```python
from build123d import *

# Parameters (mm, degrees)
SKETCH1_W           = 40
SKETCH1_H           = 60
BOSS_EXTRUDE1_DEPTH = 20
SKETCH2_R           = 15
CUT_EXTRUDE1_DEPTH  = 9
SKETCH3_R           = 2
CUT_EXTRUDE2_DEPTH  = 32
SKETCH4_W           = 15
SKETCH4_H           = 15
CUT_EXTRUDE3_DEPTH  = 9
SKETCH5_R           = 2.5
CUT_EXTRUDE4_DEPTH  = 11


with BuildPart() as part:
    # Sketch1 → Boss-Extrude1 (new body)
    with BuildSketch(Plane.XY):
        Rectangle(SKETCH1_W, SKETCH1_H)
    extrude(amount=BOSS_EXTRUDE1_DEPTH)

    # Sketch2 → Cut-Extrude1 (cut)
    with BuildSketch(Plane.XY.offset(20)):
        with Locations((0, 10.125)):
            Circle(SKETCH2_R)
    extrude(amount=-CUT_EXTRUDE1_DEPTH, mode=Mode.SUBTRACT)

    # Sketch3 → Cut-Extrude2 (cut)
    with BuildSketch(Plane.XY.offset(11)):
        with Locations((17.333333333, 26)):
            Circle(SKETCH3_R)
        with Locations((-17.333333333, 26)):
            Circle(SKETCH3_R)
        with Locations((17.333333333, -26)):
            Circle(SKETCH3_R)
        with Locations((-17.333333333, -26)):
            Circle(SKETCH3_R)
    extrude(amount=-CUT_EXTRUDE2_DEPTH, mode=Mode.SUBTRACT)

    # Sketch4 → Cut-Extrude3 (cut)
    with BuildSketch(Plane.XY.offset(20)):
        with Locations((-20, 30)):
            Rectangle(SKETCH4_W, SKETCH4_H)
        with Locations((20, 30)):
            Rectangle(SKETCH4_W, SKETCH4_H)
        with Locations((-20, -30)):
            Rectangle(SKETCH4_W, SKETCH4_H)
        with Locations((20, -30)):
            Rectangle(SKETCH4_W, SKETCH4_H)
    extrude(amount=-CUT_EXTRUDE3_DEPTH, mode=Mode.SUBTRACT)

    # Sketch5 → Cut-Extrude4 (cut)
    with BuildSketch(Plane.XY.offset(11)):
        with Locations((0, 10.125)):
            Circle(SKETCH5_R)
    extrude(amount=-CUT_EXTRUDE4_DEPTH, mode=Mode.SUBTRACT)


solid = part.part
```
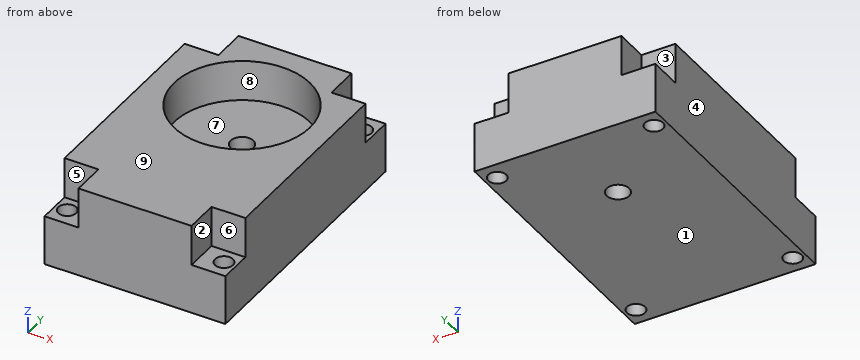
Model file for the job. Use its own axes, mm. Face numbers are marked on the shaded views. A direction names the side the tool comes from. Round coordinates to 2 decimals unless told otherwise and drop trailing zeros. Loops run counter-clockwise (first coordinate to the right, second up) from the corner with the lowest first, then second, coordinate; pieces in that order, holes last. Notation, with made-up numbers: M -21.75,11.25 L -14.75,11.25 A21 ccw -14.75,17.25 Z; hole C 77.25,-25.5 d6. An arc over 180 degrees is marked long. Put each result on its own line as item: value. Start each with the question number.
Item 1: Cut at B-B (y = 26). List the corners of the cut face in (x, z), then the cut area to 3 significant figures.
Item 2: Drill centre lines: line 1 along X through (y, z) = (-27, 1.5); line 2 along Y through (x, z) = (0, 8) (3 decimals); line 3 along Y through (x, z) = (0, 14.75) (3 decimals). Where is each one in solid material? Low to high.
Item 3: Cut at D-D (x = -17). List the corners of the cut face in (y, z), then the cut area to 3 significant figures.
Item 4: 3-axis set-ups, long thin cutter, end or side, ignore diameter. For the marked faces 1, 2, 3, 4 and 5: which of +Z, -Z, +X, -X, +Y, -Y reach the whole face in a straight line?
Item 5: Cut at A-A (x = 0). List the corners of the cut face in (y, z) (3 decimals).
Item 6: Cut at C-C (z = 7.5). List the corners of the cut face in (x, y) (3 decimals).
Item 7: Drop flat-ended pins along their axis: P1, Ø2, axis at y = 25.5, z = 17.5, coming from the -X side; P2, Ø2, axis at y = 26.5, z = 16.5, coming from the +X side; P3, Ø5, axis at x = 17.33, y = -26, coming from the +Z side. Give the stop position or say it passes through.
Item 8: Mould opens along Y. For the marked faces 6, 7, 8 and 9 say: released by +Y, released by -Y, zero draft, split by the parting line, or undercut.
Answer block:
1. outline: M -20,0 L -19.33,0 L -19.33,11 L -20,11 Z; M -15.33,0 L 15.33,0 L 15.33,11 L 12.5,11 L 12.5,20 L -12.5,20 L -12.5,11 L -15.33,11 Z; M 19.33,0 L 20,0 L 20,11 L 19.33,11 Z
1. area: 577 mm2
2. line 1: -20 to -19.07, -15.6 to 15.6, 19.07 to 20
2. line 2: -30 to 7.625, 12.625 to 30
2. line 3: -30 to -4.875, 25.125 to 30
3. outline: M -30,0 L -27.97,0 L -27.97,11 L -30,11 Z; M -24.03,0 L 24.03,0 L 24.03,11 L 22.5,11 L 22.5,20 L -22.5,20 L -22.5,11 L -24.03,11 Z; M 27.97,0 L 30,0 L 30,11 L 27.97,11 Z
3. area: 978 mm2
4. face 1: -Z, +X, -X, +Y, -Y
4. face 2: +Z, +X, -Y
4. face 3: +Z, -X, +Y
4. face 4: +Z, -Z, -X, +Y, -Y
4. face 5: +Z, -X, -Y
5. outline: M -30,0 L 7.625,0 L 7.625,11 L -4.875,11 L -4.875,20 L -30,20 Z; M 12.625,0 L 30,0 L 30,20 L 25.125,20 L 25.125,11 L 12.625,11 Z
6. outline: M -20,-30 L 20,-30 L 20,30 L -20,30 Z; hole C -17.333,-26 d4; hole C -17.333,26 d4; hole C 0,10.125 d5; hole C 17.333,-26 d4; hole C 17.333,26 d4
7. P1: x = -12.5
7. P2: x = 12.5
7. P3: z = 11
8. face 6: released by -Y
8. face 7: undercut
8. face 8: undercut
8. face 9: zero draft
